Can you work these out from the drawing? Everything is in mm from the part's minimum corner. A direction names the side the tool comes from. Coordinates: 2 decimals unless noted, no trailing zeros. Order: outer loops, then holes, each group sorted by start corner. A loop starts at its lowest first (then second) coordinate and runs counter-clockwise, first axis right, second up. Notation, with made-up numbers: M -28.5,-4 L -3.5,-4 A17 ccw -3.5,28 Z; hole C -18,-1 d3. An arc over 180 degrees is marked long. Answer as a JSON object with one key per item and string values.
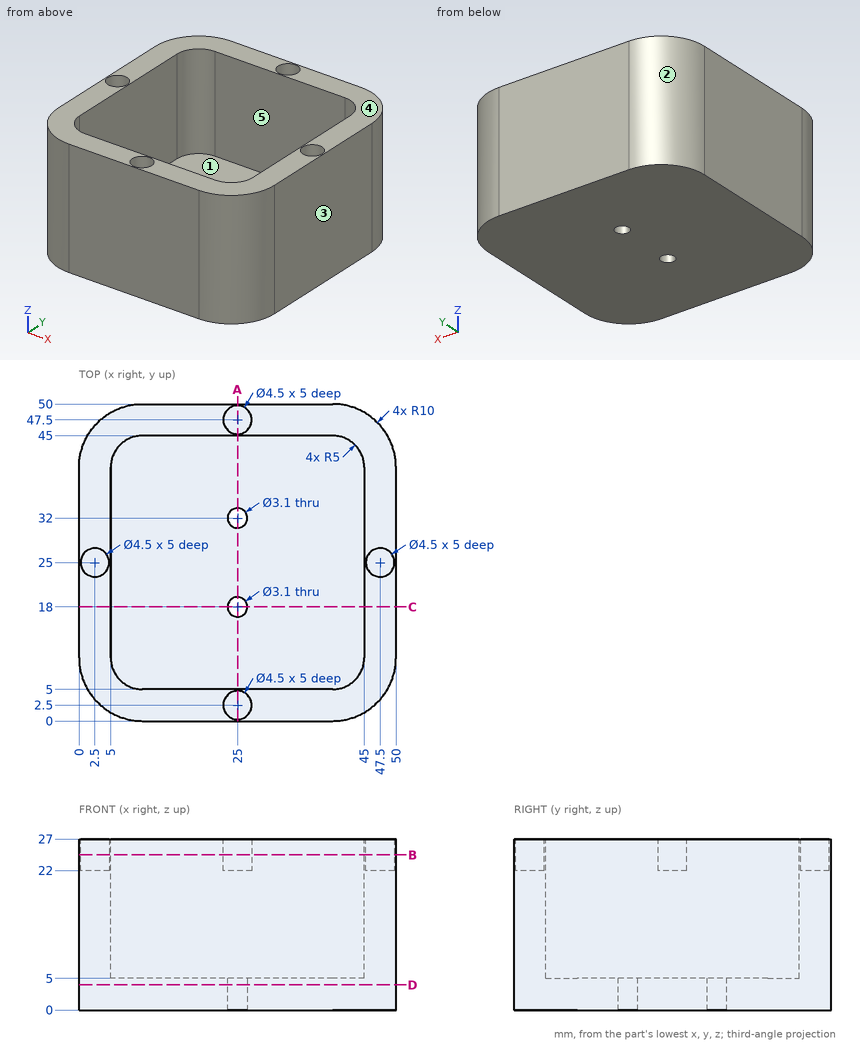
Item 1: I want a section at D-D, the plane z = 4. Write out the boundary of the cut face in (x, y).
Answers follow:
{"outline": "M 0,10 A10 ccw 10,0 L 40,0 A10 ccw 50,10 L 50,40 A10 ccw 40,50 L 10,50 A10 ccw 0,40 Z; hole C 25,18 d3.1; hole C 25,32 d3.1"}
Item 2: Which directions (+Z, -Z, +X, -X, +Y, -Y) give clear straight access to the entire face, cutting with the end or side of a thin tool? Please do the marked faces 1 and 2.
Answers follow:
{"face 1": "+Z", "face 2": "+Z, -Z, -X, +Y"}
Item 3: I want a section at A-A, the plane x = 25. Write out the boundary of the cut face in (y, z), plus the area to 3 significant figures.
Answers follow:
{"outline": "M 0,0 L 16.45,0 L 16.45,5 L 5,5 L 5,27 L 4.75,27 L 4.75,22 L 0.25,22 L 0.25,27 L 0,27 Z; M 19.55,0 L 30.45,0 L 30.45,5 L 19.55,5 Z; M 33.55,0 L 50,0 L 50,27 L 49.75,27 L 49.75,22 L 45.25,22 L 45.25,27 L 45,27 L 45,5 L 33.55,5 Z", "area": "394 mm^2"}
Item 4: I want a section at C-C, the plane y = 18. Write out the boundary of the cut face in (x, z).
Answers follow:
{"outline": "M 0,0 L 23.45,0 L 23.45,5 L 5,5 L 5,27 L 0,27 Z; M 26.55,0 L 50,0 L 50,27 L 45,27 L 45,5 L 26.55,5 Z"}
Item 5: If we mould it in two halves opening along X, with no side actions, what happens to the marked faces 3, 4 and 5? For each: pulls with the +X half, pulls with the -X half, needs draft (parallel to the pull), parting line crosses it, or undercut.
Answers follow:
{"face 3": "pulls with the +X half", "face 4": "needs draft", "face 5": "undercut"}
Item 6: I want a section at B-B, the plane z = 24.5. Write out the boundary of the cut face in (x, y).
Answers follow:
{"outline": "M 0,10 A10 ccw 10,0 L 40,0 A10 ccw 50,10 L 50,40 A10 ccw 40,50 L 10,50 A10 ccw 0,40 Z; hole C 2.5,25 d4.5; hole M 5,10 A5 ccw 10,5 L 40,5 A5 ccw 45,10 L 45,40 A5 ccw 40,45 L 10,45 A5 ccw 5,40 Z; hole C 25,2.5 d4.5; hole C 25,47.5 d4.5; hole C 47.5,25 d4.5"}
Item 7: I'm going to push flat-ended pins straight in: pin 1 (1.9 mm diameter, centred on x = 25, y = 32, fed in from -Z); pin 2 (6 mm diameter, centred on x = 31.5, y = 23, fed in from +Z); pin 3 (1.3 mm diameter, centred on x = 25.5, y = 48.5, fed in from +Z). Where does each tip first touch, or does it pass through?
Answers follow:
{"pin 1": "passes through", "pin 2": "stops at z = 5", "pin 3": "stops at z = 22"}
Item 8: Please list where these lines run through material, in increasing order: line 1 (Y direction, x = 17, z = 8.25); line 2 (Y direction, x = 25, z = 2.95).
Answers follow:
{"line 1": "y = 0 to 5, 45 to 50", "line 2": "y = 0 to 16.45, 19.55 to 30.45, 33.55 to 50"}
